Autodesk Inventor part; units mm, degrees
ref_plane "YZ Plane" through (0, 0, 0) normal (1, 0, 0) x (0, 1, 0)
ref_plane "XZ Plane" through (0, 0, 0) normal (0, 1, 0) x (-1, 0, 0)
ref_plane "XY Plane" through (0, 0, 0) normal (0, 0, 1) x (1, 0, 0)
sketch "Skizze1" plane through (0, 0, 0) normal (0, 0, 1) x (1, 0, 0)
  line L0 (0, 0) -> (130, 0)
  line L1 (130, 0) -> (130, 2.5)
  line L2 (130, 2.5) -> (70, 2.5)
  line L3 (70, 2.5) -> (55, 7.5)
  line L4 (0, 7.5) -> (0, 0)
  line L5 (-57.0949, 0) -> (91.8524, 0)
  line L6 (-94.5139, 0) -> (167.419, 0)
  line L7 (0, -1.5) -> (0, 9)
  line L8 (11, 7.5) -> (11, 6.5)
  line L9 (11, 6.5) -> (13, 6.5)
  line L10 (13, 6.5) -> (13, 7.5)
  line L11 (55, 7.5) -> (13, 7.5)
  line L12 (11, 7.5) -> (0, 7.5)
  point P0 (0, 0)
  point P1 (0, -1.5)
  point P2 (0, 9)
  dimension "d0" = 130
  dimension "d1" = 5
  dimension "d3" = 55
  dimension "d4" = 15
  dimension "d5" = 11
  dimension "d6" = 2
  dimension "d7" = 1
  dimension "d8" = 15
revolve "Umdrehung1" add sketch "Skizze1" angle 360 about axis through (-57.0949, 0, 0) along (1, 0, 0)
sketch "Skizze2" plane through (0, 0, 0) normal (0, 1, 0) x (-1, 0, 0)
  line L0 (0, 2.5) -> (-10, 2.5)
  line L1 (-10, 2.5) -> (-10, -2.5)
  line L2 (-10, -2.5) -> (0, -2.5)
  line L3 (0, -2.5) -> (0, 2.5)
  point P0 (0, 0)
  point P1 (0, 0)
  dimension "d10" = 10
  dimension "d11" = 5
extrude "Extrusion1" cut sketch "Skizze2" along normal through all both and the other way through all
sketch "Skizze3" plane through (0, 0, 0) normal (0, 0, 1) x (1, 0, 0)
  circle A0 centre (5, 0) radius 2.25
  line L0 (0, -7.0711) -> (0, 7.0711)
  point P0 (0, 0)
  point P1 (0, 0)
  dimension "d14" = 5
  dimension "d15" = 4.5
extrude "Extrusion2" cut sketch "Skizze3" along normal through all both and the other way through all
thread "Gewinde1"
properties part number "Anker"
Can you work these out from the model? Positions are in its coordinate system, mm. A direction names the side the tool comes from. Round coordinates to 2 decimals unless told otherwise and drop trailing zeros. Loops run counter-clockwise (first coordinate to the right, second up) from the corner with the lowest first, then second, coordinate; pieces in that order, holes last.
Item 1: Suppose I cut it at C-C, the plane x = 5. Write out the boundary of the cut face in (y, z), then the cut area to 3 significant figures.
Item 2: Which directions (+Z, -Z, +X, -X, +Y, -Y) give clear straight access to the entire face, cutting with the end or side of a thin tool? Please do faces 1 (the flat face through (7, -2, -2.5)), 2 (the flat face through (13, -6, 3)), 3 (the cylindrical face through (99.58, -0.54, 2.44)).
Item 3: Suppose I cut it at A-A, the plane y = 0. Write out the boundary of the cut face in (x, z), then the cut area to 3 significant figures.
Item 4: Will these pins go through, and if not, where does the flat tip stop? pin 1 Ø1.5 at (x, z) = (56.5, 0.5) entering from -Y; pin 2 Ø3 at (x, z) = (33, -3) entering from +Y; pin 3 Ø8 at (x, y) = (16, 3.5) entering from +Z; pin 4 Ø2 at (x, z) = (76, -1.5) entering from -Y.
Item 5: Please list where these lines run through material, in increasing order: L1, parallel to Y at x = 124.5, z = 0.25; L2, parallel to X at y = -5, z = 5.5; L3, parallel to Y at x = 5, z = -4.1.
Item 6: If we mould it in two halves opening along X, with no side actions, what happens to faces 4 (the flat face through (11, -6, 3)), 5 (the flat face through (0, 0, 4)), 6 (the cylindrical face through (33.706, -7.493, -0.33))? For each: +X half, -X half, draft (parallel to the pull), parting line (faces both ways), or undercut.
Item 7: Suppose I cut it at B-B, the plane z = 0. Write out the boundary of the cut face in (x, y), then the cut area to 3 significant figures.
Item 8: Suppose I cut it at D-D, the plane x = 100.5. Write out the boundary of the cut face in (y, z), then the cut area to 3 significant figures.
Reported:
1. outline: (-7.07, -2.5) arc R7.5 ccw to (-2.25, -7.15) - (-2.25, -2.5) - close; (-7.07, 2.5) - (-2.25, 2.5) - (-2.25, 7.15) arc R7.5 ccw to start; (2.25, -7.15) arc R7.5 ccw to (7.07, -2.5) - (2.25, -2.5) - close; (2.25, 2.5) - (7.07, 2.5) arc R7.5 ccw to (2.25, 7.15) - close
1. area: 59.2 mm2
2. face 1: -X, +Y, -Y
2. face 2: none
2. face 3: +X
3. outline: (0, -7.5) - (2.75, -7.5) - (2.75, -2.5) - (0, -2.5) - close; (0, 2.5) - (2.75, 2.5) - (2.75, 7.5) - (0, 7.5) - close; (7.25, -7.5) - (11, -7.5) - (11, -6.5) - (13, -6.5) - (13, -7.5) - (55, -7.5) - (70, -2.5) - (130, -2.5) - (130, 2.5) - (70, 2.5) - (55, 7.5) - (13, 7.5) - (13, 6.5) - (11, 6.5) - (11, 7.5) - (7.25, 7.5) - (7.25, 2.5) - (10, 2.5) - (10, -2.5) - (7.25, -2.5) - close
3. area: 1,180 mm2
4. pin 1: stops at y = -7.24
4. pin 2: stops at y = 7.35
4. pin 3: stops at z = 7.5
4. pin 4: stops at y = -2.45
5. L1: y = -2.49 to 2.49
5. L2: x = 0 to 11, 13 to 55.2
5. L3: y = -6.28 to -2.25, 2.25 to 6.28
6. face 4: undercut
6. face 5: -X half
6. face 6: draft
7. outline: (10, -7.5) - (11, -7.5) - (11, -6.5) - (13, -6.5) - (13, -7.5) - (55, -7.5) - (70, -2.5) - (130, -2.5) - (130, 2.5) - (70, 2.5) - (55, 7.5) - (13, 7.5) - (13, 6.5) - (11, 6.5) - (11, 7.5) - (10, 7.5) - close
7. area: 1,120 mm2
8. outline: circle Ø5 at (0, 0)
8. area: 19.6 mm2
